```python
from build123d import *

# Parameters (mm, degrees)
SKETCH1_W           = 67.4
SKETCH1_H           = 67.4
BOSS_EXTRUDE1_DEPTH = 1.2
BOSS_EXTRUDE2_START = 12.85
SKETCH2_W           = 69.8
SKETCH2_H           = 69.8
SKETCH2_W_2         = 67.4
SKETCH2_H_2         = 67.4
BOSS_EXTRUDE2_DEPTH = 12.85
BOSS_EXTRUDE3_DEPTH = 10.7


with BuildPart() as part:
    # Sketch1 → Boss-Extrude1 (new body)
    with BuildSketch(Plane(origin=(0, 0, 0), x_dir=(1, 0, 0), z_dir=(0, 1, 0))):
        with BuildLine():
            Line((-22.840165497, 18.147363877), (-10.340165497, 18.147363877))
            Line((-10.340165497, 18.147363877), (-10.340165497, 24.147363877))
            Line((-10.340165497, 24.147363877), (41.409834503, 24.147363877))
            Line((41.409834503, 24.147363877), (41.409834503, 18.147363877))
            Line((41.409834503, 18.147363877), (53.909834503, 18.147363877))
            ThreePointArc((53.909834503, 18.147363877), (54.616941284, 17.854470658), (54.909834503, 17.147363877))
            Line((54.909834503, 17.147363877), (54.909834503, -59.602636123))
            ThreePointArc((54.909834503, -59.602636123), (54.616941284, -60.309742904), (53.909834503, -60.602636123))
            Line((53.909834503, -60.602636123), (-22.840165497, -60.602636123))
            ThreePointArc((-22.840165497, -60.602636123), (-23.547272279, -60.309742904), (-23.840165497, -59.602636123))
            Line((-23.840165497, -59.602636123), (-23.840165497, 17.147363877))
            ThreePointArc((-23.840165497, 17.147363877), (-23.547272279, 17.854470658), (-22.840165497, 18.147363877))
        make_face()
        with Locations((15.534834503, -21.227636123)):
            Rectangle(SKETCH1_W, SKETCH1_H, mode=Mode.SUBTRACT)
    extrude(amount=BOSS_EXTRUDE1_DEPTH)

    # Sketch2 → Boss-Extrude2 (add)
    # profile 1 of 2: a face of its own
    with BuildSketch(Plane.XZ.offset(BOSS_EXTRUDE2_START)):
        with BuildLine():
            Line((41.409834503, -24.147363877), (-10.340165497, -24.147363877))
            Line((-10.340165497, -24.147363877), (-10.340165497, -18.147363877))
            Line((-10.340165497, -18.147363877), (-22.840165497, -18.147363877))
            ThreePointArc((-22.840165497, -18.147363877), (-23.547272279, -17.854470658), (-23.840165497, -17.147363877))
            Line((-23.840165497, -17.147363877), (-23.840165497, 59.602636123))
            ThreePointArc((-23.840165497, 59.602636123), (-23.547272279, 60.309742904), (-22.840165497, 60.602636123))
            Line((-22.840165497, 60.602636123), (53.909834503, 60.602636123))
            ThreePointArc((53.909834503, 60.602636123), (54.616941284, 60.309742904), (54.909834503, 59.602636123))
            Line((54.909834503, 59.602636123), (54.909834503, -17.147363877))
            ThreePointArc((54.909834503, -17.147363877), (54.616941284, -17.854470658), (53.909834503, -18.147363877))
            Line((53.909834503, -18.147363877), (41.409834503, -18.147363877))
            Line((41.409834503, -18.147363877), (41.409834503, -24.147363877))
        make_face()
        Polygon((40.209834503, -22.947363877), (-9.140165497, -22.947363877), (-9.140165497, -16.947363877), (-22.640165497, -16.947363877), (-22.640165497, 59.402636123), (53.709834503, 59.402636123), (53.709834503, -16.947363877), (40.209834503, -16.947363877), align=None, mode=Mode.SUBTRACT)
    # profile 2 of 2: a face of its own
    with BuildSketch(Plane.XZ.offset(BOSS_EXTRUDE2_START)):
        with Locations((15.534834503, 21.227636123)):
            Rectangle(SKETCH2_W, SKETCH2_H)
        with Locations((15.534834503, 21.227636123)):
            Rectangle(SKETCH2_W_2, SKETCH2_H_2, mode=Mode.SUBTRACT)
    extrude(amount=-BOSS_EXTRUDE2_DEPTH)

    # Sketch3 → Boss-Extrude3 (add)
    with BuildSketch(Plane.XZ.offset(12.85)):
        Polygon((-9.140165497, -22.947363877), (-10.340165497, -22.947363877), (-10.340165497, -24.147363877), (41.409834503, -24.147363877), (41.409834503, -22.947363877), align=None)
    extrude(amount=BOSS_EXTRUDE3_DEPTH)


solid = part.part
```
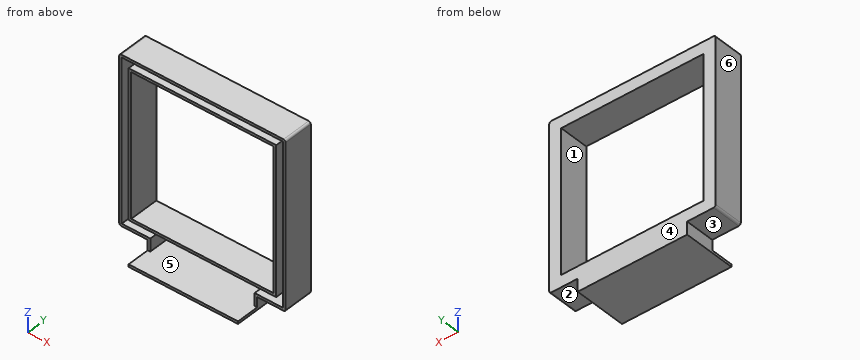
The listing builds one solid part. Answer for the finished solid, in the listing's coordinates (mm). Face numbers are marked on the shaded views. A direction names the side the tool comes from. Coordinates: 2 decimals unless noted, no trailing zeros. Loops run counter-clockwise (first coordinate to the right, second up) from the corner with the lowest first, then second, coordinate; pieces in that order, holes last. Notation, with made-up numbers: (-38.75, -30) - (-25.75, -30) arc R31 ccw to (-25.75, 7) - close; hole circle Ø11 at (25.5, 81). An arc over 180 degrees is marked (long way). Use a Markdown table: item, result. Add a question column.
1) The part is cut by section C-C, the plane z = -1. Give the vertices of the cut face in (x, y), and give its area (3 significant figures).
2) The mould has two halves that part along X. Classify the marked faces 4, 5 and 6: released by +X, released by -X, zero draft, split by the parting line, or undercut.
3) Given pin 1 (5 mm diameter, centred on y = -9, z = -20, fed in from +X); pin 2 (1.8 mm diameter, centred on y = -9, z = -19.5, fed in from -X); pin 3 (5 mm diameter, centred on y = -4.5, z = -18.5, fed in from +X), each flat-ended and moving along its own axis, determine where each tip first touches the part or whether it passes through.
4) For the marked faces 1, 2 and 3, determine the directions among +Z, -Z, +X, -X, +Y, -Y from which every point of the face is accessible in a straight line to the end or side of a thin tool.
5) The part is cut by section B-B, the plane x = 25. Give the vertices of the cut face in (y, z).
6) The part is cut by section D-D, the plane y = -17.25. Give the vertices of the cut face in (x, z).
7) The part is cut by section A-A, the plane y = -10. Give the vertices of the cut face in (x, z), and give its area (3 significant figures).
8) Find the intervals of material crossed by line 1 (X direction, y = -10.5, z = -13); line 2 (X direction, y = -1, z = 51); line 3 (Z direction, x = 29, y = -4.25), in increasing order.
Here are the results:
| question | item | result |
|---|---|---|
| 1 | outline | (-23.84, -12.85) - (-22.64, -12.85) - (-22.64, 0) - (-19.37, 0) - (-19.37, -12.85) - (-18.17, -12.85) - (-18.17, 1.2) - (-23.84, 1.2) - close; (49.23, -12.85) - (50.43, -12.85) - (50.43, 0) - (53.71, 0) - (53.71, -12.85) - (54.91, -12.85) - (54.91, 1.2) - (49.23, 1.2) - close |
| 1 | area | 75.3 mm^2 |
| 2 | face 4 | zero draft |
| 2 | face 5 | undercut |
| 2 | face 6 | released by -X |
| 3 | pin 1 | stops at x = 54.85 |
| 3 | pin 2 | stops at x = -10.34 |
| 3 | pin 3 | stops at x = 54.91 |
| 4 | face 1 | +Y, -Y |
| 4 | face 2 | -Z, +X, +Y, -Y |
| 4 | face 3 | -Z, -X, +Y, -Y |
| 5 | outline | (-23.55, -24.15) - (1.2, -24.15) - (1.2, -12.47) - (-12.85, -12.47) - (-12.85, -13.67) - (0, -13.67) - (0, -22.95) - (-23.55, -22.95) - close; (-12.85, 54.93) - (1.2, 54.93) - (1.2, 60.6) - (-12.85, 60.6) - (-12.85, 59.4) - (0, 59.4) - (0, 56.13) - (-12.85, 56.13) - close |
| 6 | outline | (-10.34, -24.15) - (41.41, -24.15) - (41.41, -22.95) - (-10.34, -22.95) - close |
| 7 | outline | (-23.84, -17.15) arc R1 ccw to (-22.84, -18.15) - (-10.34, -18.15) - (-10.34, -24.15) - (41.41, -24.15) - (41.41, -18.15) - (53.91, -18.15) arc R1 ccw to (54.91, -17.15) - (54.91, 59.6) arc R1 ccw to (53.91, 60.6) - (-22.84, 60.6) arc R1 ccw to (-23.84, 59.6) - close; (-19.37, -13.67) - (50.43, -13.67) - (50.43, 56.13) - (-19.37, 56.13) - close; hole (-22.64, -16.95) - (-9.14, -16.95) - (-9.14, -22.95) - (40.21, -22.95) - (40.21, -16.95) - (53.71, -16.95) - (53.71, 59.4) - (-22.64, 59.4) - close; hole (-18.17, -12.47) - (49.23, -12.47) - (49.23, 54.93) - (-18.17, 54.93) - close |
| 7 | area | 715 mm^2 |
| 8 | line 1 | x = -23.84 to -22.64, -19.37 to 50.43, 53.71 to 54.91 |
| 8 | line 2 | x = -23.84 to -22.64, -19.37 to -18.17, 49.23 to 50.43, 53.71 to 54.91 |
| 8 | line 3 | z = -24.15 to -22.95, -13.67 to -12.47, 54.93 to 56.13, 59.4 to 60.6 |
